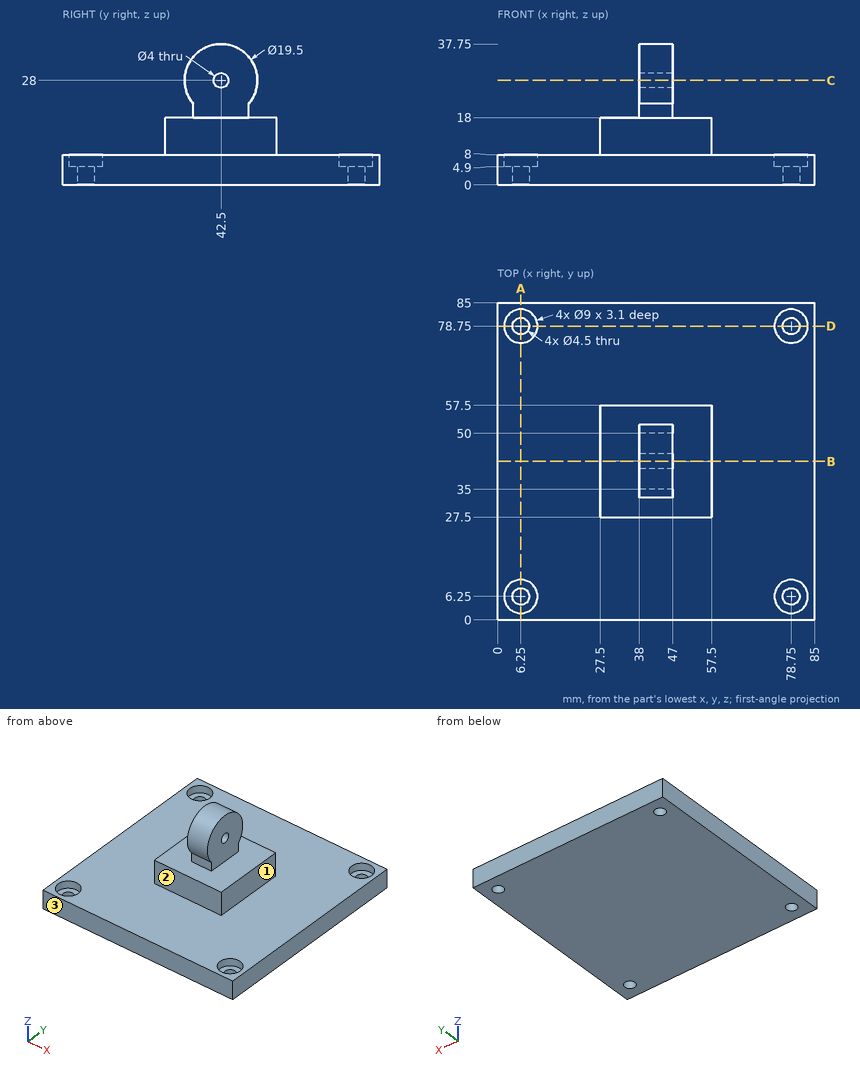
Input: dimensioned drawing with shaded views. Units: mm. Origin: part minimum x, y, z. A direction names the side the tool comes from. Give positions to 0.01 mm unless a question says otherwise; leave off trailing zeros. Order: outer loops, then holes, each group sorted by start corner. A loop starts at its lowest first (then second) coordinate and runs counter-clockwise, first axis right, second up. Notation, with made-up numbers: (-15.5, 13) -> (10.5, 13) arc R17 ccw to (10.5, 32) -> close; hole circle Ø4 at (-1.75, 54). An arc over 180 degrees is marked (long way). Answer as a JSON object with one key per item and string values.
Q1. Access query for the marked faces 1, 2 and 3. Directions: +Z, -Z, +X, -X, +Y, -Y. A direction counts if a zero-diameter tool reaches every point of the face in a straight line with its end or side. Return the directions, or none.
Entries:
{"face 1": "+Z, +X, +Y, -Y", "face 2": "+Z, +X, -X, -Y", "face 3": "+Z, -Z, +X, -X, -Y"}
Q2. Section C-C (z = 28). Output: boundary loops of the cut face in (x, y).
Entries:
{"outline": "(38, 32.75) -> (47, 32.75) -> (47, 40.5) -> (38, 40.5) -> close; (38, 44.5) -> (47, 44.5) -> (47, 52.25) -> (38, 52.25) -> close"}
Q3. First-contact query: pin 1 (4.5 mm diameter, centred on y = 42.5, z = 28, fed in from +X); pin 2 (3 mm diameter, centred on y = 39, z = 13.5, fed in from -X); pin 3 (8 mm diameter, centred on x = 42.5, z = 13, fed in from -Y). Flat tips, straight axial feed; report the tip coordinate or a pass-through.
Entries:
{"pin 1": "stops at x = 47", "pin 2": "stops at x = 27.5", "pin 3": "stops at y = 27.5"}
Q4. Section A-A (x = 6.25). Output: boundary loops of the cut face in (y, z).
Entries:
{"outline": "(0, 0) -> (4, 0) -> (4, 4.9) -> (1.75, 4.9) -> (1.75, 8) -> (0, 8) -> close; (8.5, 0) -> (76.5, 0) -> (76.5, 4.9) -> (74.25, 4.9) -> (74.25, 8) -> (10.75, 8) -> (10.75, 4.9) -> (8.5, 4.9) -> close; (81, 0) -> (85, 0) -> (85, 8) -> (83.25, 8) -> (83.25, 4.9) -> (81, 4.9) -> close"}
Q5. Material intervals for probe 1 along X at (y, z) = (78.75, 2.85); probe 2 along Y at (x, z) = (42, 28), sorted ascending.
Entries:
{"probe 1": "x = 0 to 4, 8.5 to 76.5, 81 to 85", "probe 2": "y = 32.75 to 40.5, 44.5 to 52.25"}
Q6. Section B-B (y = 42.5). Output: boundary loops of the cut face in (x, z), plus the area to 3 significant figures.
Entries:
{"outline": "(0, 0) -> (85, 0) -> (85, 8) -> (57.5, 8) -> (57.5, 18) -> (47, 18) -> (47, 26) -> (38, 26) -> (38, 18) -> (27.5, 18) -> (27.5, 8) -> (0, 8) -> close; (38, 30) -> (47, 30) -> (47, 37.75) -> (38, 37.75) -> close", "area": "1,120 mm^2"}
